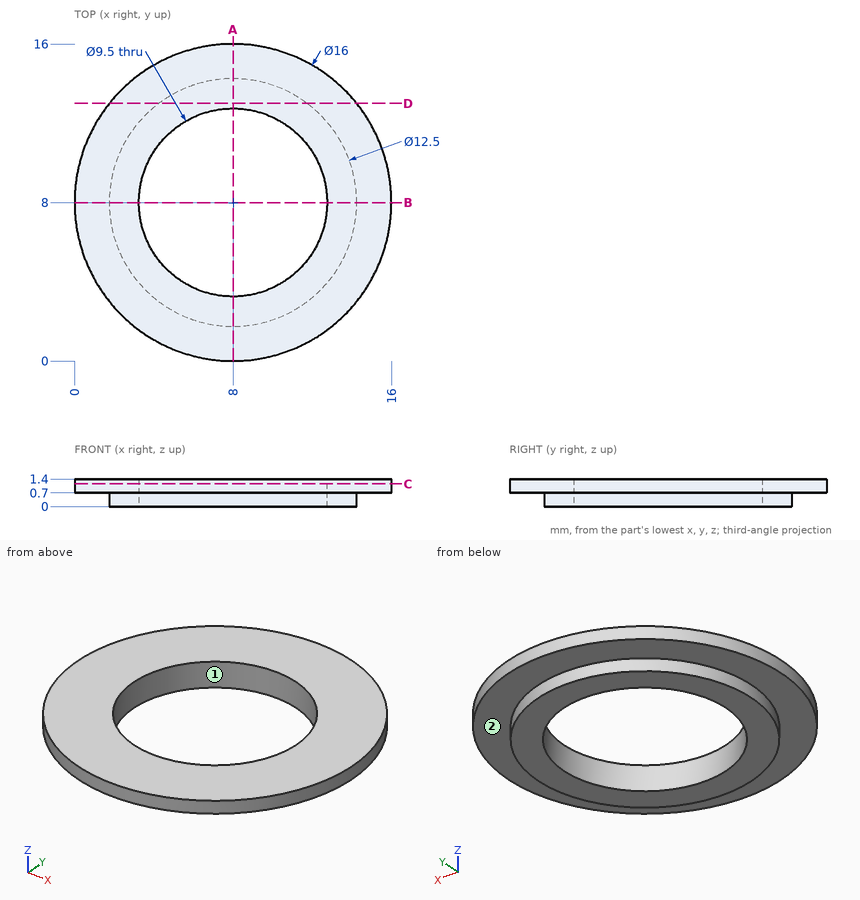
For this review, use the dimensioned drawing (mm, ordinates from the lowest corner) and the shaded views. Round coordinates to 2 decimals unless told otherwise and drop trailing zeros. Write each loop counter-clockwise with the first axis right and the second up, starting at its lowest first coordinate (ties: lowest second). Pieces come first, ordered by that corner, then holes. Notation, with made-up numbers: M -13,65.25 L 29,65.25 A25 cw 29,77.25 Z; hole C 42,-5 d8. An arc over 180 degrees is marked long. Answer as CSV lines item,"result". Start each with the question number.
Q1. Wall thickness on line 1 along Y through (x, z) = (8, 0.55); line 2 along Z through (x, y) = (4.25, 14); line 3 along Y through (x, z) = (8, 0.85): over which ranges is each line inside the solid? List them lowest first.
Q2. The part is to be moulded in two halves that separate along Y. For the marked faces 1 and 2, say which applies: +Y half, -Y half, draft (parallel to the pull), parting line (faces both ways), or undercut.
Q3. Consider section C-C, the plane z = 1.15. Give the boundary of the cut face in (x, y), then the cut area to 3 significant figures.
Q4. Consider section A-A, the plane x = 8. Give the boundary of the cut face in (y, z).
Q5. Consider section D-D, the plane y = 13. Give the boundary of the cut face in (x, z) (3 decimals), then the cut area to 3 significant figures.
Result set:
1,line 1,"y = 1.75 to 3.25, 12.75 to 14.25"
1,line 2,"z = 0.7 to 1.4"
1,line 3,"y = 0 to 3.25, 12.75 to 16"
2,face 1,"undercut"
2,face 2,"draft"
3,outline,"C 8,8 d16; hole C 8,8 d9.5"
3,area,"130 mm²"
4,outline,"M 0,0.7 L 1.75,0.7 L 1.75,0 L 3.25,0 L 3.25,1.4 L 0,1.4 Z; M 12.75,0 L 14.25,0 L 14.25,0.7 L 16,0.7 L 16,1.4 L 12.75,1.4 Z"
5,outline,"M 1.755,0.7 L 4.25,0.7 L 4.25,0 L 11.75,0 L 11.75,0.7 L 14.245,0.7 L 14.245,1.4 L 1.755,1.4 Z"
5,area,"14.0 mm²"
